Geometry: final body of the model. Coordinates: model frame, mm. A direction names the side the tool comes from. Round coordinates to 2 decimals unless told otherwise and drop trailing zeros. Write each loop counter-clockwise with the first axis right and the second up, starting at its lowest first coordinate (ties: lowest second). Pieces come first, ordered by that corner, then holes. Notation, with made-up numbers: M 15.25,62.5 L 23.25,62.5 A21 cw 23.25,89.5 Z; hole C -30,58 d5. An arc over 180 degrees is marked long. Use one line per item in the form item = value. Start each with the question number.
from build123d import *

# Parameters (mm, degrees)
F1_DEPTH  = 2
F3_R      = 3.5
F3_R_2    = 1
F5_DEPTH  = 5
F2_W      = 2
F2_H      = 13
F2_H_2    = 18.4
F2_H_3    = 10
F6_DEPTH  = 20.5
F8_DEPTH  = 1
F4_W      = 21
F4_H      = 41
F9_DEPTH  = 25
F10_DEPTH = 25
F11_SIZE2 = 1.5
F11_SIZE  = 1.5
F4_W_2    = 8
F4_H_2    = 10
F12_DEPTH = 25


with BuildPart() as f1:
    # F0 (on Top) → F1 (new body)
    with BuildSketch(Plane.XY):
        with BuildLine():
            Line((-50.9090909091, 30), (-50.9090909091, -30))
            ThreePointArc((-50.9090909091, -30), (59.0909090909, 0), (-50.9090909091, 30))
        make_face()
    extrude(amount=F1_DEPTH)

    # F3 (on face) → F5 (join)
    with BuildSketch(Plane.XY.offset(2)):
        with Locations((0, -50.0909090909)):
            Circle(F3_R)
        with Locations((0, -50.0909090909)):
            Circle(F3_R_2, mode=Mode.SUBTRACT)
        with Locations((0, 50.0909090909)):
            Circle(F3_R)
        with Locations((0, 50.0909090909)):
            Circle(F3_R_2, mode=Mode.SUBTRACT)
        with Locations((50.0909090909, 0)):
            Circle(F3_R)
        with Locations((50.0909090909, 0)):
            Circle(F3_R_2, mode=Mode.SUBTRACT)
    extrude(amount=F5_DEPTH)

    # F2 (on face) → F6 (join)
    with BuildSketch(Plane.XY.offset(2)):
        with BuildLine():
            ThreePointArc((-48.9090909091, 29.4494945164), (57.0909090909, 0), (-48.9090909091, -29.4494945164))
            Line((-48.9090909091, -29.4494945164), (-48.9090909091, -22.0505054836))
            Line((-48.9090909091, -22.0505054836), (-50.9090909091, -22.0505054836))
            Line((-50.9090909091, -22.0505054836), (-50.9090909091, -30))
            ThreePointArc((-50.9090909091, -30), (59.0909090909, 0), (-50.9090909091, 30))
            Line((-50.9090909091, 30), (-50.9090909091, 19.3494945164))
            Line((-50.9090909091, 19.3494945164), (-48.9090909091, 19.3494945164))
            Line((-48.9090909091, 19.3494945164), (-48.9090909091, 29.4494945164))
        make_face()
        with Locations((-49.9090909091, 12.8494945164)):
            Rectangle(F2_W, F2_H)
        with Locations((-49.9090909091, -2.8505054836)):
            Rectangle(F2_W, F2_H_2)
        with Locations((-49.9090909091, -17.0505054836)):
            Rectangle(F2_W, F2_H_3)
    extrude(amount=F6_DEPTH)

    # F7 (on face) → F8 (join)
    with BuildSketch(Plane.XY.offset(22.5)):
        with BuildLine():
            Line((-49.9567093584, 29.4494945164), (-49.9567093584, -29.4494945164))
            ThreePointArc((-49.9567093584, -29.4494945164), (57.9909090909, 0), (-49.9567093584, 29.4494945164))
        make_face()
        with BuildLine():
            ThreePointArc((-48.9090909091, 29.4494945164), (57.0909090909, 0), (-48.9090909091, -29.4494945164))
            Line((-48.9090909091, -29.4494945164), (-48.9090909091, 29.4494945164))
        make_face(mode=Mode.SUBTRACT)
    extrude(amount=F8_DEPTH)

    # F4 (on face) → F9 (cut)
    with BuildSketch(Plane.XY.offset(2)):
        with Locations((32.0909090909, -10)):
            Rectangle(F4_W, F4_H)
    extrude(amount=-F9_DEPTH, mode=Mode.SUBTRACT)

    # F3 (on face) → F10 (cut)
    with BuildSketch(Plane.XY.offset(2)):
        with Locations((0, 50.0909090909)):
            Circle(F3_R_2)
        with Locations((50.0909090909, 0)):
            Circle(F3_R_2)
        with Locations((0, -50.0909090909)):
            Circle(F3_R_2)
    extrude(amount=-F10_DEPTH, mode=Mode.SUBTRACT)

    # F11
    f11_edges = [f1.edges().sort_by_distance(p)[0] for p in [
        (-1, -50.090909, 0),
        (49.090909, 0, 0),
        (-1, 50.090909, 0),
    ]]
    chamfer(f11_edges, length=F11_SIZE, length2=F11_SIZE2)

    # F4 (on face) → F12 (cut)
    with BuildSketch(Plane.XY.offset(2)):
        with Locations((12.5909090909, -8)):
            Rectangle(F4_W_2, F4_H_2)
    extrude(amount=-F12_DEPTH, mode=Mode.SUBTRACT)


solid = f1.part
1. Section query C-C (z = 9). Return loops of the section in (x, y).
2. Contact query for flat-ended pins moving along their axis: pin 1 (5.5 mm diameter, centred on x = 1, y = -50, fed in from +Z); pin 2 (2 mm diameter, centred on x = 13, z = 1, fed in from -Y); pin 3 (1 mm diameter, centred on x = 31, z = 1, fed in from -Y). Output: stop coordinate, or through.
3. Section query D-D (y = 40.5). Return loops of the section in (x, z), then the cut area to 3 significant figures.
4. Pull-direction query (X, two-part tool) for faces 1 (the face through (32.4, 48.4, 22.5)), 2 (the face through (-0.46, -46.62, 4.46)), 3 (the face through (-50.909, 0, 11)); classes: released by +X, released by -X, zero draft, split by the parting line, or undercut.
5. Section query A-A (y = -10.5). Return loops of the section in (x, z).
6. Set-up query: faces 4 (the face through (57.053, 2.077, 12.599)), 5 (the face through (59.05, -2.16, 11.09)). Return all of +Z, -Z, +X, -X, +Y, -Y with unobstructed straight access to the full face (end or side cutting, diameter ignored); none if empty.
7. Ray query, probe 1 along Y at (x, z) = (0, 1.85); probe 2 along Y at (x, z) = (0, 14); probe 3 along Z at (x, y) = (-13.5, 28). Return the intervals inside material, ascending.
8. Section query B-B (x = 13). Return loops of the section in (y, z) (3 decimals).
Checks:
q1.outline = M -50.91,-30 A59.09 ccw long -50.91,30 Z; hole M -48.91,-29.45 A57.09 ccw long -48.91,29.45 Z
q2.pin_1 = 7
q2.pin_2 = -57.86
q2.pin_3 = -50.61
q3.outline = M -43.03,0 L 43.03,0 L 43.03,22.5 L 41.51,22.5 L 41.51,23.5 L 40.24,23.5 L 40.24,2 L -40.24,2 L -40.24,23.5 L -41.51,23.5 L -41.51,22.5 L -43.03,22.5 Z
q3.area = 289 mm^2
q4.face_1 = zero draft
q4.face_2 = undercut
q4.face_3 = released by -X
q5.outline = M -50.91,0 L 8.59,0 L 8.59,2 L -48.91,2 L -48.91,23.5 L -49.96,23.5 L -49.96,22.5 L -50.91,22.5 Z; M 16.59,0 L 21.59,0 L 21.59,2 L 16.59,2 Z; M 42.59,0 L 58.15,0 L 58.15,22.5 L 57.03,22.5 L 57.03,23.5 L 56.12,23.5 L 56.12,2 L 42.59,2 Z
q6.face_4 = +Z
q6.face_5 = +Z, -Z
q7.probe_1 = -59.09 to -51.09, -49.09 to 49.09, 51.09 to 59.09
q7.probe_2 = -59.09 to -57.09, 57.09 to 59.09
q7.probe_3 = 0 to 2
q8.outline = M -57.643,0 L -13,0 L -13,2 L -55.591,2 L -55.591,23.5 L -56.515,23.5 L -56.515,22.5 L -57.643,22.5 Z; M -3,0 L 57.643,0 L 57.643,22.5 L 56.515,22.5 L 56.515,23.5 L 55.591,23.5 L 55.591,2 L -3,2 Z
